Design review of the part built by this model. Coordinates are the model's own, in mm. A direction names the side the tool comes from. Round coordinates to 2 decimals unless told otherwise and drop trailing zeros. Order: outer loops, then holes, each group sorted by start corner. A loop starts at its lowest first (then second) coordinate and runs counter-clockwise, first axis right, second up. Notation, with made-up numbers: M -27,12.25 L -16,12.25 A21 ccw -16,43.25 Z; hole C 34,-8.75 d2. An arc over 180 degrees is marked long. Use a Markdown table: item, result. Add a question column.
(1) Take a section at D-D (y = -16). Write out the cut boundary in (x, z).
(2) The part is to be moulded in two halves that separate along Y. For faces 3 (the face through (-9, 0.95, 2)), 4 (the face through (0, -4, 3.81)), 5 (the face through (-0.074, -15.495, 1.878)), 6 (the face through (-9, -0.95, 2)), say which applies: released by +Y, released by -Y, zero draft, split by the parting line, or undercut.
(3) Machinability: for faces 1 (the face through (18.248, 4.467, 1.878)), 2 (the face through (-3.4, 0, 1.9)), which of the approach directions +Z, -Z, +X, -X, +Y, -Y give a long, thin tool a straight path to every point of the face, cutting with its end or side? Answer none if there is none.
(4) Take a section at C-C (x = 1). Write out the cut boundary in (y, z).
(5) Take a section at B-B (z = 2.5). Write out the cut boundary in (x, y), then the cut area to 3 significant figures.
(6) Take a section at A-A (y = 0). Write out the cut boundary in (x, z), then the cut area to 3 significant figures.
(7) To check wall thickness, follow probe 1 along Y at (x, z) = (0, 1.25); probe 2 along X at (y, z) = (-0.5, 3.05); probe 3 along Y at (x, z) = (-4, 1.7). State the ranges of each line that lie inside material, in increasing order. Write a range as from..to.
```python
from build123d import *

# Parameters (mm, degrees)
BOSS_EXTRUDE1_DEPTH = 3.81
SKETCH4_R           = 1.984375
CUT_EXTRUDE2_DEPTH  = 27.977511323


with BuildPart() as part:
    # Sketch1 → Boss-Extrude1 (new body)
    with BuildSketch(Plane.XY):
        with BuildLine():
            Line((17.43361247, 4.7625), (-17.43361247, 4.7625))
            ThreePointArc((-17.43361247, 4.7625), (-18.238621898, 4.474772784), (-18.678870503, 3.741964286))
            ThreePointArc((-18.678870503, 3.741964286), (-15.796789426, -10.647250529), (-3.540477767, -18.718106667))
            ThreePointArc((-3.540477767, -18.718106667), (0, -15.494), (3.540477767, -18.718106667))
            ThreePointArc((3.540477767, -18.718106667), (15.796789426, -10.647250529), (18.678870503, 3.741964286))
            ThreePointArc((18.678870503, 3.741964286), (18.238621898, 4.474772784), (17.43361247, 4.7625))
        make_face()
    extrude(amount=BOSS_EXTRUDE1_DEPTH)

    # Sketch4 → Cut-Extrude2 (cut, through all)
    with BuildSketch(Plane.XY.offset(3.81)):
        Circle(SKETCH4_R)
        with BuildLine():
            Line((-14.350000002, 0.95), (-4.35, 0.95))
            ThreePointArc((-4.35, 0.95), (-3.4, 0), (-4.35, -0.95))
            Line((-4.35, -0.95), (-14.350000002, -0.95))
            ThreePointArc((-14.350000002, -0.95), (-15.300000002, 0), (-14.350000002, 0.95))
        make_face()
        with BuildLine():
            Line((4.35, 0.95), (14.350000002, 0.95))
            ThreePointArc((14.350000002, 0.95), (15.300000002, 0), (14.350000002, -0.95))
            Line((14.350000002, -0.95), (4.35, -0.95))
            ThreePointArc((4.35, -0.95), (3.4, 0), (4.35, 0.95))
        make_face()
    extrude(amount=-CUT_EXTRUDE2_DEPTH, mode=Mode.SUBTRACT)


solid = part.part
```
Verdict:
| question | item | result |
|---|---|---|
| 1 | outline | M -10.34,0 L -1.83,0 L -1.83,3.81 L -10.34,3.81 Z; M 1.83,0 L 10.34,0 L 10.34,3.81 L 1.83,3.81 Z |
| 2 | face 3 | undercut |
| 2 | face 4 | zero draft |
| 2 | face 5 | released by -Y |
| 2 | face 6 | undercut |
| 3 | face 1 | +Z, -Z, +X, +Y |
| 3 | face 2 | +Z, -Z |
| 4 | outline | M -15.64,0 L -1.71,0 L -1.71,3.81 L -15.64,3.81 Z; M 1.71,0 L 4.76,0 L 4.76,3.81 L 1.71,3.81 Z |
| 5 | outline | M -18.68,3.74 A19.05 ccw -3.54,-18.72 A3.56 cw 3.54,-18.72 A19.05 ccw 18.68,3.74 A1.27 ccw 17.43,4.76 L -17.43,4.76 A1.27 ccw Z; hole M -14.35,-0.95 L -4.35,-0.95 A0.95 ccw -4.35,0.95 L -14.35,0.95 A0.95 ccw Z; hole C 0,0 d3.97; hole M 4.35,-0.95 L 14.35,-0.95 A0.95 ccw 14.35,0.95 L 4.35,0.95 A0.95 ccw Z |
| 5 | area | 674 mm^2 |
| 6 | outline | M -19.05,0 L -15.3,0 L -15.3,3.81 L -19.05,3.81 Z; M -3.4,0 L -1.98,0 L -1.98,3.81 L -3.4,3.81 Z; M 1.98,0 L 3.4,0 L 3.4,3.81 L 1.98,3.81 Z; M 15.3,0 L 19.05,0 L 19.05,3.81 L 15.3,3.81 Z |
| 6 | area | 39.4 mm^2 |
| 7 | probe 1 | y = -15.49..-1.98, 1.98..4.76 |
| 7 | probe 2 | x = -19.04..-15.16, -3.54..-1.92, 1.92..3.54, 15.16..19.04 |
| 7 | probe 3 | y = -18.63..-0.88, 0.88..4.76 |
